Here's the drawing with two shaded views (mm, measured from the low corner). I have some questions. Round coordinates to 2 decimals unless told otherwise and drop trailing zeros. Loops run counter-clockwise (first coordinate to the right, second up) from the corner with the lowest first, then second, coordinate; pieces in that order, holes last. Notation, with made-up numbers: M -37.75,36 L 3.25,36 A17 ccw 3.25,48 Z; hole C 1,26.5 d5. An arc over 180 degrees is marked long. Answer as CSV lines item,"result".
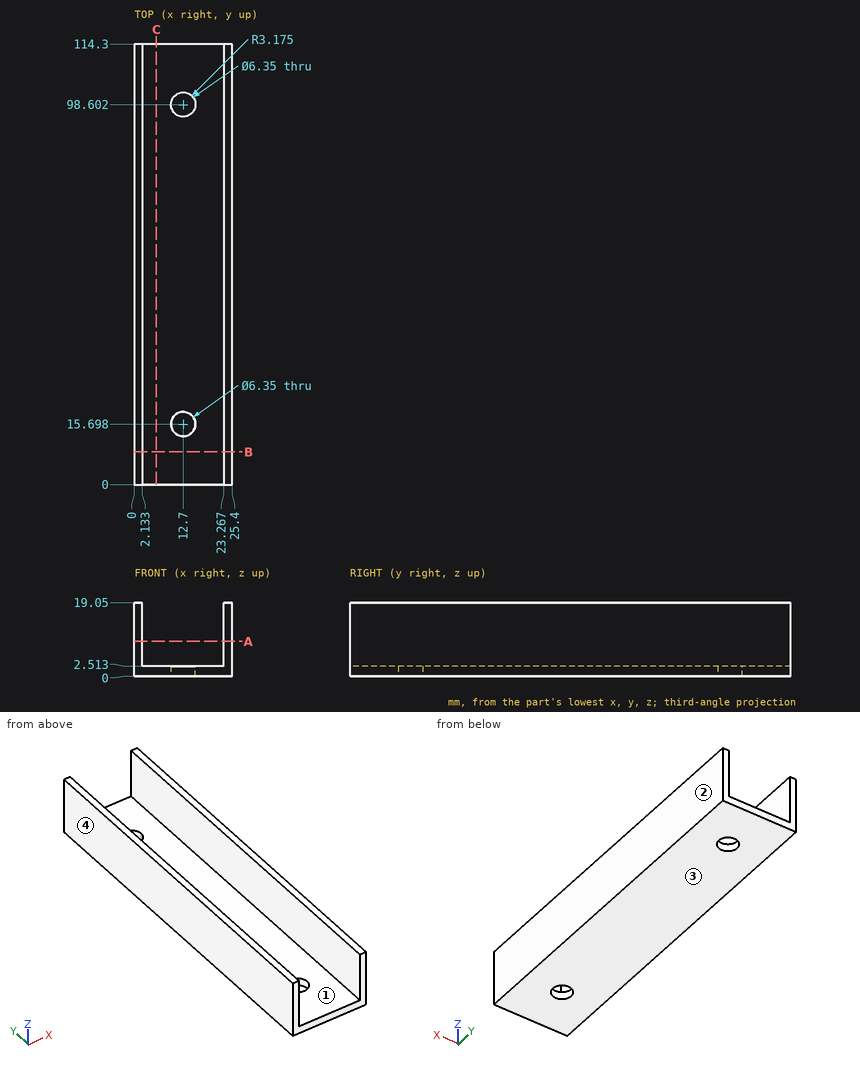
1. We'd pull the mould along X, two halves only. Please class the marked faces 1, 2, 3 and 4: pulls with the +X half, pulls with the -X half, needs draft (parallel to the pull), parting line crosses it, or undercut.
Evaluation:
face 1,"undercut"
face 2,"pulls with the +X half"
face 3,"needs draft"
face 4,"pulls with the -X half"
2. I want a section at C-C, the plane x = 5.75. Please give me the cut outline in (y, z).
Evaluation:
outline,"M 0,0 L 114.3,0 L 114.3,2.51 L 0,2.51 Z"
3. I want a section at A-A, the plane z = 9. Please give me the cut outline in (x, y).
Evaluation:
outline,"M 0,0 L 2.13,0 L 2.13,114.3 L 0,114.3 Z; M 23.27,0 L 25.4,0 L 25.4,114.3 L 23.27,114.3 Z"
4. If I drill on line 1 (Y direction, x = 12.7, z = 1.55); line 2 (X direction, y = 110, z = 10.5); line 3 (Z direction, x = 16.75, y = 7), over which ranges is the centre line in solid material (lowest first)? Write a range as [from, to].
Evaluation:
line 1,"y = [0, 12.52], [18.87, 95.43], [101.78, 114.3]"
line 2,"x = [0, 2.13], [23.27, 25.4]"
line 3,"z = [0, 2.51]"
5. I want a section at B-B, the plane y = 8.5. Please give me the cut outline in (x, z).
Evaluation:
outline,"M 0,0 L 25.4,0 L 25.4,19.05 L 23.27,19.05 L 23.27,2.51 L 2.13,2.51 L 2.13,19.05 L 0,19.05 Z"
6. For P1, Ø10, axis at x = 12.7, y = 98.6, coming from the +Z side, with a flat end and sliding along its axis, tell me the tip position at first contact or that it passes through.
Evaluation:
P1,"stops at z = 2.51"
